For this review, take the finished solid that the model builds, in its own axes (mm). A direction names the side the tool comes from. Coordinates: 2 decimals unless noted, no trailing zeros. Order: outer loops, then holes, each group sorted by start corner. A loop starts at its lowest first (then second) coordinate and runs counter-clockwise, first axis right, second up. Notation, with made-up numbers: (36, 3.25) -> (51, 3.25) arc R28 ccw to (51, 41.25) -> close; hole circle Ø8 at (50.5, 73). An arc over 180 degrees is marked (long way). Return JSON: item names as keys, results as strings. Group by question number.
Item 1: Take a section at B-B (x = 17). Write out the cut boundary in (y, z), then the cut area to 3 significant figures.
Item 2: For line 1 along X through (y, z) = (2.25, -1.5); line 2 along Z through (x, y) = (-20.5, 0.75); line 3 along X through (y, z) = (2.8, 16.5), list the stretches that pass through material, from the lowest coordinate up.
Item 3: Insertion check: pin 1 (2 mm diameter, centred on x = 35, y = 2, fed in from -Z); pin 2 (1.2 mm diameter, centred on x = -36.5, y = 2, fed in from -Z); pin 3 (2 mm diameter, centred on y = 1.5, z = -4.5, fed in from -X); pin 4 (6 mm diameter, centred on x = 24, z = -25.5, fed in from +Y). Each pin has a flat end and moves straight along its axis. Give the tip position at first contact, or say it passes through.
Item 4: Take a section at C-C (z = 38.5). Write out the cut boundary in (x, y), then the cut area to 3 significant figures.
Item 5: Take a section at A-A (x = 0). Write out the cut boundary in (y, z).
Item 6: Draft analysis for pull direction Z (two halves, no side actions). For faces 3 (the flat face through (3, 4.064, 27)), 4 (the flat face through (36, 2, 0)), state which applies: +Z half, -Z half, draft (parallel to the pull), parting line (faces both ways), or undercut.
Item 7: Take a section at D-D (y = 1.45). Count the separate pieces of the cut face and the enclosed holes in it, then the cut area to 3 significant figures.
Item 8: Machinability: for faces 1 (the flat face through (3, 0, 27)), 2 (the flat face through (-17.97, 2.06, 31.126)), which of the approach directions +Z, -Z, +X, -X, +Y, -Y give a long, thin tool a straight path to every point of the face, cutting with its end or side? Answer none if there is none.
```python
from build123d import *

# Parameters (mm, degrees)
SKETCH1_R           = 44.45
SKETCH1_R_2         = 26.67
BOSS_EXTRUDE1_DEPTH = 4.064
CUT_EXTRUDE1_REACH  = 64.993
CIRPATTERN1_COUNT   = 9


with BuildPart() as part:
    # Sketch1 → Boss-Extrude1 (new body)
    with BuildSketch(Plane(origin=(0, 0, 0), x_dir=(1, 0, 0), z_dir=(0, 1, 0))):
        with Locations(Location((0, 0, 0), (0, 0, 90))):
            Circle(SKETCH1_R)
        with Locations(Location((0, 0, 0), (0, 0, 90))):
            Circle(SKETCH1_R_2, mode=Mode.SUBTRACT)
    extrude(amount=BOSS_EXTRUDE1_DEPTH)

    # Sketch2 → Cut-Extrude1 (cut, up to next)
    with BuildSketch(Plane(origin=(0, 4.064, 0), x_dir=(1, 0, 0), z_dir=(0, 1, 0)), mode=Mode.PRIVATE) as cut_extrude1_sk1:
        with BuildLine():
            Line((-28.760847548, 0), (-42.922177943, 0))
            ThreePointArc((-42.922177943, 0), (-42.270093615, 7.453357981), (-40.333653882, 14.680249452))
            Line((-40.333653882, 14.680249452), (-27.026356208, 9.8367892))
            ThreePointArc((-27.026356208, 9.8367892), (-28.323905648, 4.994268765), (-28.760847548, 0))
        make_face()
    cut_extrude1_tool1 = extrude(cut_extrude1_sk1.sketch, amount=-CUT_EXTRUDE1_REACH, mode=Mode.PRIVATE) & part.part
    cut_extrude1 = cut_extrude1_tool1.solids().sort_by_distance((-35.574933, 4.064, -6.27282))[0]
    add(cut_extrude1, mode=Mode.SUBTRACT)

    # CirPattern1: Cut-Extrude1 ×9 about axis
    cirpattern1_axis = Axis((0, 0, 0), (0, 1, 0))
    for i in range(1, CIRPATTERN1_COUNT):
        add(cut_extrude1.rotate(cirpattern1_axis, i * 360 / CIRPATTERN1_COUNT), mode=Mode.SUBTRACT)


solid = part.part
```
Findings below:
{
 "1": {"outline": "(0, -41.07) -> (4.06, -41.07) -> (4.06, -29.44) -> (0, -29.44) -> close; (0, -23.2) -> (4.06, -23.2) -> (4.06, -20.55) -> (0, -20.55) -> close; (0, 20.55) -> (4.06, 20.55) -> (4.06, 29.44) -> (0, 29.44) -> close; (0, 39.41) -> (4.06, 39.41) -> (4.06, 41.07) -> (0, 41.07) -> close", "area": "101 mm2"},
 "2": {"line 1": "x = -44.42 to -42.9, -28.72 to -26.63, 26.63 to 28.72, 42.9 to 44.42", "line 2": "z = -39.44 to -35.51, -20.17 to -17.06, 17.06 to 35.51, 37.71 to 39.44", "line 3": "x = -41.27 to -39.62, -23.56 to -20.95, 20.95 to 23.56, 39.62 to 41.27"},
 "3": {"pin 1": "stops at z = -28.63", "pin 2": "stops at z = -26.21", "pin 3": "stops at x = -44.31", "pin 4": "passes through"},
 "4": {"outline": "(-22.22, 0) -> (-18.98, 0) -> (-18.98, 4.06) -> (-22.22, 4.06) -> close; (-6.79, 0) -> (6.79, 0) -> (6.79, 4.06) -> (-6.79, 4.06) -> close; (18.98, 0) -> (22.22, 0) -> (22.22, 4.06) -> (18.98, 4.06) -> close", "area": "81.5 mm2"},
 "5": {"outline": "(0, -44.45) -> (4.06, -44.45) -> (4.06, -42.92) -> (0, -42.92) -> close; (0, -28.76) -> (4.06, -28.76) -> (4.06, -26.67) -> (0, -26.67) -> close; (0, 26.67) -> (4.06, 26.67) -> (4.06, 44.45) -> (0, 44.45) -> close"},
 "6": {"face 3": "draft", "face 4": "undercut"},
 "7": {"separate pieces": "1", "enclosed holes": "10", "area": "2,380 mm2"},
 "8": {"face 1": "+Z, -Z, +X, -X, -Y", "face 2": "+Y, -Y"}
}
